Check sheet for the modelled part. Datum: model origin and axes. Units: mm. A direction names the side the tool comes from. Give positions to 0.01 mm unless a question says otherwise; leave off trailing zeros. Loops run counter-clockwise (first coordinate to the right, second up) from the corner with the lowest first, then second, coordinate; pieces in that order, holes last. Notation, with made-up numbers: M 36,26 L 55,26 A34 cw 55,60 Z; hole C 33,7.5 d5. An arc over 180 degrees is marked long. Put each result on its own line as item: value. Start each with the question number.
Solid Edge part; units mm, degrees
sketch "Sketch1" plane through (0, 0, 0) normal (0, 0, 1) x (1, 0, 0)
  line L0 (-17.0658, 2.676) -> (-26.3732, 16.1486)
  arc A0 (-26.3732, 23.6514) -> (-26.3732, 16.1486) centre (-20.9429, 19.9) ccw
  line L1 (-17.0658, 37.124) -> (-26.3732, 23.6514)
  arc A1 (-17.0658, 37.124) -> (-8.8647, 38.9694) centre (-11.9647, 33.6) cw
  line L2 (12.906, 26.4) -> (-8.8647, 38.9694)
  line L3 (22.4644, 26.4) -> (12.906, 26.4)
  arc A2 (22.4644, 13.4) -> (22.4644, 26.4) centre (22.4644, 19.9) ccw
  line L4 (12.906, 13.4) -> (22.4644, 13.4)
  line L5 (4.5154, 8.5556) -> (12.906, 13.4)
  line L6 (1.4843, 6.8056) -> (4.5154, 8.5556)
  line L7 (-8.8647, 0.8306) -> (1.4843, 6.8056)
  arc A3 (-17.0658, 2.676) -> (-8.8647, 0.8306) centre (-11.9647, 6.2) ccw
  circle A4 centre (-20.7647, 19.9) radius 2.2
  circle A5 centre (22.4644, 19.9) radius 2.2
extrude "Protrusion1" add sketch "Sketch1" along normal blind 3
sketch "Sketch2" plane through (-1.5893, 19.9, 3) normal (0, 0, 1) x (-0.5, 0.866, 0)
  circle A0 centre (-6.6768, 15.8354) radius 3.7
  circle A1 centre (17.0523, 2.1354) radius 3.7
  circle A2 centre (-6.6768, -11.5646) radius 3.7
extrude "ExtrudedCutout_1" cut sketch "Sketch2" against normal blind 80.9131
sketch "Sketch3" plane through (0.7107, 19.9, 3) normal (0, 0, 1) x (-0.866, 0.5, 0)
  circle A0 centre (4.144, 2.3732) radius 4.5
extrude "Cutout1" cut sketch "Sketch3" against normal blind 107.7727
Q1. Section check C-C, the plane z = 2.2. Record the cut outline in (x, y).
Q2. Depth check by flat-ended pin: P1, Ø1.5, axis at x = 17.5, z = 1, coming from the +Y side; P2, Ø1.5, axis at y = 11.5, z = 2, coming from the -X side. Enter the tip coordinate at first touch or a pass-through.
Q3. Thickness scan on line 1 along X through (y, z) = (17, 1); line 2 along Y through (x, z) = (12, 2.8); line 3 along Y through (x, z) = (-4.5, 0.65). Record the ranges inside material, lowest first. Write a range as [from, to].
Q4. Mould release check, pull along X, two halves, no side actions. Record for faces 1 (the face through (-14.9, 31.35, 1.52)), 2 (the face through (2.17, 32.6, 1.48)), 3 (the face through (-13.389, 39.634, 1.479)), 4 (the face through (1, 20, 0)): pulls with the +X half, pulls with the -X half, needs draft (parallel to the pull), parting line crosses it, or undercut.
Q5. Section check D-D, the plane x = 21. Record the cut outline in (y, z).
Q6. Section check A-A, the plane y = 36. Record the cut outline in (x, z).
Q7. Section check B-B, the plane x = -12.5. Record the cut outline in (y, z).
Q8. Access from +Z, -Z, +X, -X, +Y, -Y to the whole of each face (thin tool, end or side, straight path). Record for faces 5 (the face through (18, 13.4, 1)), 6 (the face through (-21.654, 9.318, 1.479)), 7 (the face through (18, 26.4, 1)).
Found:
1. outline: M -26.37,16.15 L -17.07,2.68 A6.2 ccw -8.86,0.83 L 1.48,6.81 L 4.52,8.56 L 12.91,13.4 L 22.46,13.4 A6.5 ccw 22.46,26.4 L 12.91,26.4 L -8.86,38.97 A6.2 ccw -17.07,37.12 L -26.37,23.65 A6.6 ccw Z; hole C -20.76,19.9 d4.4; hole C -11.96,6.2 d7.4; hole C -11.96,33.6 d7.4; hole C -4.06,19.92 d9; hole C 11.76,19.9 d7.4; hole C 22.46,19.9 d4.4
2. P1: stops at y = 26.4
2. P2: stops at x = -23.68
3. line 1: x = [-26.87, -7.49], [-0.64, 9.47], [14.06, 28.28]
3. line 2: y = [12.88, 16.21], [23.59, 26.92]
3. line 3: y = [3.35, 15.44], [24.4, 36.45]
4. face 1: undercut
4. face 2: pulls with the +X half
4. face 3: parting line crosses it
4. face 4: needs draft
5. outline: M 13.4,0 L 18.26,0 L 18.26,3 L 13.4,3 Z; M 21.54,0 L 26.4,0 L 26.4,3 L 21.54,3 Z
6. outline: M -17.84,0 L -14.78,0 L -14.78,3 L -17.84,3 Z; M -9.15,0 L -3.72,0 L -3.72,3 L -9.15,3 Z
7. outline: M 0.02,0 L 2.54,0 L 2.54,3 L 0.02,3 Z; M 9.86,0 L 29.94,0 L 29.94,3 L 9.86,3 Z; M 37.26,0 L 39.78,0 L 39.78,3 L 37.26,3 Z
8. face 5: +Z, -Z, +X, -Y
8. face 6: +Z, -Z, -X, -Y
8. face 7: +Z, -Z, +X, +Y
